Could you check a few things on this drawing? It's one solid part, dimensions in mm from its lowest x, y, z. Coordinates: 2 decimals unless noted, no trailing zeros. Order: outer loops, then holes, each group sorted by start corner. A loop starts at its lowest first (then second) coordinate and runs counter-clockwise, first axis right, second up.
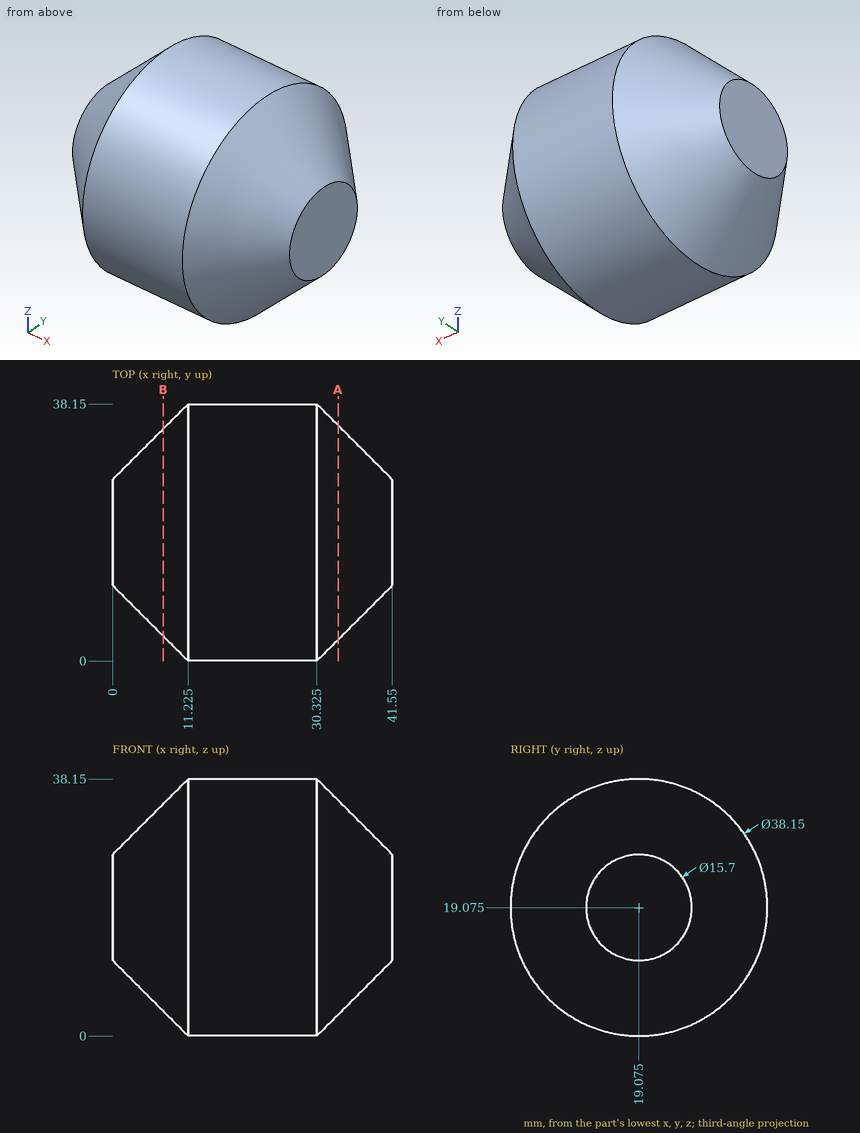
1. Please list where these lines run through material, in increasing order: probe 1 along Z at (x, y) = (23, 11); probe 2 along Y at (x, z) = (15, 13.5); probe 3 along Y at (x, z) = (30.5, 4).
Completed:
probe 1: z = 1.79 to 36.36
probe 2: y = 0.83 to 37.32
probe 3: y = 7.68 to 30.47
2. Imagine slicing it at B-B on x = 7.5. Please give me the cut outline in (y, z) (3 decimals).
Completed:
outline: circle Ø30.7 at (19.075, 19.075)
3. I'm going to push flat-ended pins straight in: pin 1 (8 mm diameter, centred on x = 33, y = 5, fed in from -Z); pin 2 (2 mm diameter, centred on y = 28.5, z = 15.5, fed in from +X); pin 3 (6 mm diameter, centred on x = 16, y = 5, fed in from +Z). Where does each tip first touch, or does it pass through?
Completed:
pin 1: stops at z = 3.56
pin 2: stops at x = 40.32
pin 3: stops at z = 34.61
4. Imagine slicing it at A-A on x = 33.5. Please give me the cut outline in (y, z) (3 decimals).
Completed:
outline: circle Ø31.8 at (19.075, 19.075)
